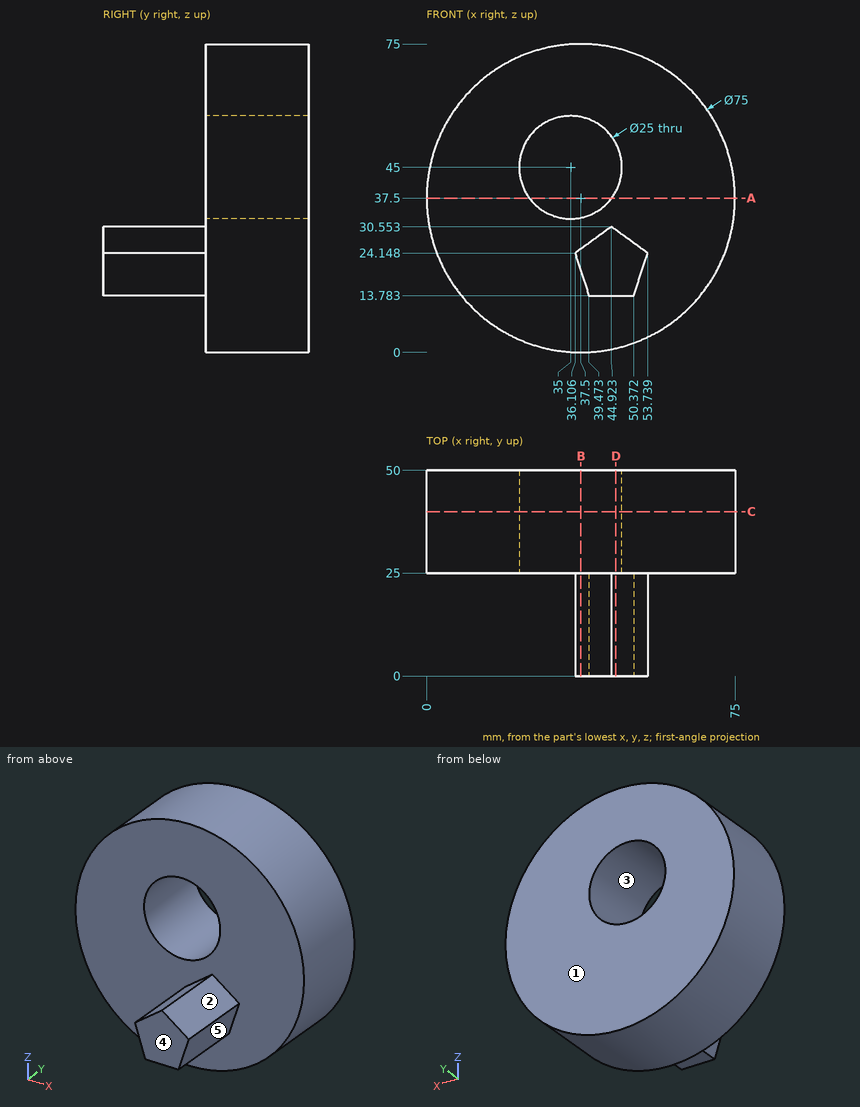
The figure shows three views and two pictorial views of one solid part (mm, origin at its lowest corner). Answer the questions. A direction names the side the tool comes from. Give positions to 0.01 mm unless a question says otherwise; leave off trailing zeros. Order: outer loops, then holes, each group sorted by start corner. A loop starts at its lowest first (then second) coordinate and runs counter-clockwise, first axis right, second up. Notation, with made-up numbers: (-15.5, -2) -> (9.5, -2) arc R27 cw to (9.5, 33) -> close; hole circle Ø1 at (85, 89.25). An arc over 180 degrees is marked (long way). Answer as a JSON object with one key per item and string values. Group by question number.
Item 1: A tool of negligible diameter and unlimited length cuts with its end or side. For the marked faces 4 and 5, from which of +Z, -Z, +X, -X, +Y, -Y can it reach the whole face along a straight path? Write none if from no direction.
Item 2: The part is cut by section D-D on x = 46. Write down the section's boundary in (y, z).
Item 3: Flat-ended cylindrical pins translate along their axes: pin 1 (4 mm diameter, centred on y = 39, z = 65, fed in from +X) (1 decimal); pin 2 (1.5 mm diameter, centred on x = 34, y = 23, fed in from -Z); pin 3 (12 mm diameter, centred on x = 38, z = 34.5, fed in from +Y); pin 4 (8 mm diameter, centred on x = 40, y = 24, fed in from +Z). Find the tip coordinate at first contact, or state that the pin passes through.
Item 4: The part is cut by section C-C on y = 40. Write down the section's boundary in (x, z), and give its area (3 significant figures).
Item 5: Consider L1, parallel to Y at x = 10, z = 55; L2, parallel to Z at x = 38.5, y = 41.5; L3, parallel to Z at x = 35, y = 42. Determine where each line is inside the solid, lowest interval first. Write a range as from..to.
Item 6: The part is cut by section A-A on z = 37.5. Write down the section's boundary in (x, y), and give its area (4 significant figures).
Item 7: Determine the mould class of the marked faces 1, 2 and 3 for opening direction X: pulls with the +X half, pulls with the -X half, needs draft (parallel to the pull), parting line crosses it, or undercut.
Item 8: The part is cut by section B-B on x = 37.5. Write down the section's boundary in (y, z), and give its area (4 significant figures).
Result set:
{
 "1": {"face 4": "+Z, -Z, +X, -X, -Y", "face 5": "-Z, +X, -Y"},
 "2": {"outline": "(0, 13.78) -> (25, 13.78) -> (25, 0.98) -> (50, 0.98) -> (50, 39.06) -> (25, 39.06) -> (25, 29.77) -> (0, 29.77) -> close; (25, 50.94) -> (50, 50.94) -> (50, 74.02) -> (25, 74.02) -> close"},
 "3": {"pin 1": "x = 65", "pin 2": "through", "pin 3": "y = 50", "pin 4": "z = 75"},
 "4": {"outline": "circle Ø75 at (37.5, 37.5); hole circle Ø25 at (35, 45)", "area": "3,930 mm²"},
 "5": {"L1": "25..50", "L2": "0.01..33, 57..74.99", "L3": "0.08..32.5, 57.5..74.92"},
 "6": {"outline": "(0, 25) -> (25, 25) -> (25, 50) -> (0, 50) -> close; (45, 25) -> (75, 25) -> (75, 50) -> (45, 50) -> close", "area": "1,375 mm²"},
 "7": {"face 1": "needs draft", "face 2": "pulls with the +X half", "face 3": "undercut"},
 "8": {"outline": "(0, 19.86) -> (25, 19.86) -> (25, 0) -> (50, 0) -> (50, 32.75) -> (25, 32.75) -> (25, 25.16) -> (0, 25.16) -> close; (25, 57.25) -> (50, 57.25) -> (50, 75) -> (25, 75) -> close", "area": "1,395 mm²"}
}
